Check sheet for the modelled part. Datum: model origin and axes. Units: mm. A direction names the side the tool comes from. Round coordinates to 2 decimals unless told otherwise and drop trailing zeros. Write each loop counter-clockwise with the first axis right and the second up, starting at its lowest first coordinate (ties: lowest second). Pieces come first, ordered by that corner, then holes. Notation, with made-up numbers: (43, -20.5) -> (64, -20.5) arc R26 cw to (64, 3.5) -> close; hole circle Ø9 at (-28, -11). An arc over 180 degrees is marked (long way). One line per item, written item: value.
from build123d import *

# Parameters (mm, degrees)
EXTRUDE_1_DEPTH     = 16
CUT_EXTRUDE_1_DEPTH = 50
EXTRUDE_2_DEPTH     = 28.5
SKETCH_4_R          = 4.5
CUT_EXTRUDE_2_DEPTH = 28.5
EXTRUDE_3_DEPTH     = 50
EXTRUDE_START       = 4
SKETCH_6_R          = 4.5
EXTRUDE_4_DEPTH     = 4
CUT_EXTRUDE_3_DEPTH = 60
CHAMFER_1_SIZE      = 1


with BuildPart() as part:
    # 草图1 → 凸台-拉伸1 (new, symmetric)
    with BuildSketch(Plane.XY):
        with BuildLine():
            Line((-17, -12.990381057), (-17, -66.86388681))
            Line((-17, -66.86388681), (-20.5, -66.86388681))
            Line((-20.5, -66.86388681), (-20.5, -12.990381057))
            ThreePointArc((-20.5, -12.990381057), (-17.809307341, -9.210736327), (-13.357142857, -10.51602276))
            ThreePointArc((-13.357142857, -10.51602276), (0, -17), (13.357142857, -10.51602276))
            ThreePointArc((13.357142857, -10.51602276), (17.809307341, -9.210736327), (20.5, -12.990381057))
            Line((20.5, -12.990381057), (20.5, -66.86388681))
            Line((20.5, -66.86388681), (17, -66.86388681))
            Line((17, -66.86388681), (17, -12.990381057))
            ThreePointArc((17, -12.990381057), (16.663663418, -12.517925466), (16.107142857, -12.68108627))
            ThreePointArc((16.107142857, -12.68108627), (0, -20.5), (-16.107142857, -12.68108627))
            ThreePointArc((-16.107142857, -12.68108627), (-16.663663418, -12.517925466), (-17, -12.990381057))
        make_face()
    extrude(amount=EXTRUDE_1_DEPTH, both=True)

    # 草图2 → 切除-拉伸1 (cut, symmetric)
    with BuildSketch(Plane(origin=(0, 0, 0), x_dir=(0, 0, -1), z_dir=(1, 0, 0))):
        Polygon((16, -60.748653355), (-16, -56.251346645), (-16, -66.86388681), (16, -66.86388681), align=None)
    extrude(amount=CUT_EXTRUDE_1_DEPTH, both=True, mode=Mode.SUBTRACT)

    # 草图3 → 凸台-拉伸2 (add)
    with BuildSketch(Plane.ZY.offset(20.5)):
        Polygon((-16, -60.748653355), (16, -56.251346645), (16, -52.716950141), (-16, -57.214256851), align=None)
    extrude_2 = extrude(amount=EXTRUDE_2_DEPTH)

    # 镜向1: 凸台-拉伸2 across plane
    add(extrude_2.mirror(Plane(origin=(0, 0, 0), x_dir=(0, 0, 1), z_dir=(1, 0, 0))))

    # 草图4 → 切除-拉伸2 (cut)
    with BuildSketch(Plane(origin=(0, -53.900966366, 7.575286804), x_dir=(1, 0, 0), z_dir=(0, 0.9902680687415715, -0.13917310096005808))):
        with Locations(Location((40.5, 7.649733485, 0), (0, 0, 270))):
            Circle(SKETCH_4_R)
        with BuildLine():
            Line((-36, 10.149733485), (-36, 5.149733485))
            ThreePointArc((-36, 5.149733485), (-40.5, 0.649733485), (-45, 5.149733485))
            Line((-45, 5.149733485), (-45, 10.149733485))
            ThreePointArc((-45, 10.149733485), (-40.5, 14.649733485), (-36, 10.149733485))
        make_face()
    extrude(amount=-CUT_EXTRUDE_2_DEPTH, mode=Mode.SUBTRACT)

    # 草图7 → 切除-拉伸3 (cut, symmetric)
    with BuildSketch(Plane(origin=(0, 0, 0), x_dir=(0, 0, -1), z_dir=(1, 0, 0))):
        Polygon((16, -60.748653355), (-16, -56.251346645), (-16, 0), (16, 0), align=None)
    extrude(amount=CUT_EXTRUDE_3_DEPTH, both=True, mode=Mode.SUBTRACT)


with BuildPart() as body_2:
    # 草图5 → 凸台-拉伸3 (new, symmetric)
    with BuildSketch(Plane(origin=(0, 0, 0), x_dir=(0, 0, -1), z_dir=(1, 0, 0))):
        Polygon((-16, -56.251346645), (16, -60.748653355), (16, -72.998653355), (-16, -72.998653355), align=None)
    extrude(amount=EXTRUDE_3_DEPTH, both=True)

    # 草图6 → 凸台-拉伸4 (add)
    with BuildSketch(Plane(origin=(0, -57.366904606, 8.062392658), x_dir=(1, 0, 0), z_dir=(0, 0.9902680687415714, -0.13917310096005842)).offset(EXTRUDE_START)):
        with Locations(Location((40.5, 7.649733485, 0), (0, 0, 90))):
            Circle(SKETCH_6_R)
        with BuildLine():
            Line((-36, 5.149733485), (-36, 10.149733485))
            ThreePointArc((-36, 10.149733485), (-40.5, 14.649733485), (-45, 10.149733485))
            Line((-45, 10.149733485), (-45, 5.149733485))
            ThreePointArc((-45, 5.149733485), (-40.5, 0.649733485), (-36, 5.149733485))
        make_face()
    extrude(amount=-EXTRUDE_4_DEPTH)

    # 倒角1
    chamfer_1_edges = [body_2.edges().sort_by_distance(p)[0] for p in [
        (-40.5, -55.444681169, -7.001463032),
        (-45, -54.470469462, -0.06958655),
        (-40.5, -53.496257755, 6.862289931),
        (-36, -54.470469462, -0.06958655),
        (40.5, -53.844190507, 4.386619759),
    ]]
    chamfer(chamfer_1_edges, length=CHAMFER_1_SIZE)


solid = body_2.part
Item 1: Sectioned sample at A-A (x = -13). Enter the section's corners in (y, z).
Result set:
outline: (-73, -16) -> (-60.75, -16) -> (-56.25, 16) -> (-73, 16) -> close
Item 2: Depth check by flat-ended pin: pin 1 (6 mm diameter, centred on x = -13.5, z = 4, fed in from +Y); pin 2 (1.8 mm diameter, centred on y = -56, z = -1, fed in from +X); pin 3 (8 mm diameter, centred on x = -19, z = -3.5, fed in from +Y). Enter the tip coordinate at first touch or a pass-through.
Result set:
pin 1: y = -57.52
pin 2: x = 44.99
pin 3: y = -58.43
Item 3: Release check for a two-part mould opening along Z. For faces 1 (the flat face through (-36, -57, 0)), 2 (the cylindrical face through (-40.401, -57.899, -6.655)), 3 (the cylindrical face through (-40.599, -55.951, 7.206)) record: pulls with the +Z half, pulls with the -Z half, needs draft (parallel to the pull), parting line crosses it, or undercut.
Result set:
face 1: needs draft
face 2: pulls with the -Z half
face 3: undercut
Item 4: Sectioned sample at B-B (z = 10.5). Enter the section's corners in (x, y).
Result set:
outline: (-50, -73) -> (50, -73) -> (50, -57.02) -> (-50, -57.02) -> close
Item 5: Tool access check on faces 4 (the flat face through (1, -72.999, 0)), 5 (the flat face through (-36.51, -54.95, 0.03)), 6 (the flat face through (-45, -57, 0)). Record the directions out of +Z, -Z, +X, -X, +Y, -Y that give a thin tool (end or side, any length) a straight path to the whole face; none if there is none.
Result set:
face 4: +Z, -Z, +X, -X, -Y
face 5: -Z, +Y
face 6: -Z, -X, +Y
Item 6: Material ranges on line 1 along X through (y, z) = (-56, -1); line 2 along X through (y, z) = (-56.5, 5); line 3 along Y through (x, z) = (12.5, 5), recorded low to high.
Result set:
line 1: -45 to -36, 36.15 to 44.85
line 2: -44.4 to -36.6
line 3: -73 to -57.8
